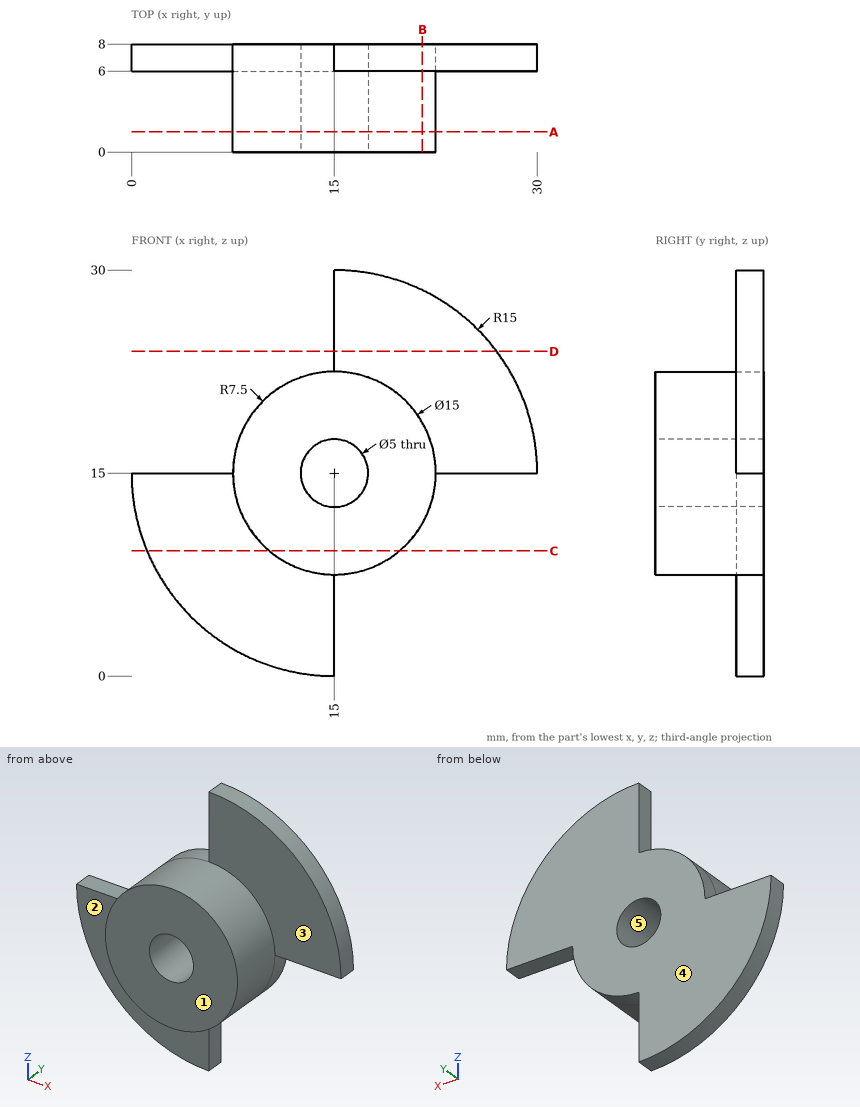
For this review, use the dimensioned drawing (mm, ordinates from the lowest corner) and the shaded views. A direction names the side the tool comes from. Coordinates: 2 decimals unless noted, no trailing zeros. Order: outer loops, then holes, each group sorted by start corner. A loop starts at its lowest first (then second) coordinate and runs counter-clockwise, first axis right, second up. Notation, with made-up numbers: (71.25, -23) - (79.25, -23) arc R26 cw to (79.25, 3) - close; hole circle Ø7 at (-18.75, 6.5). An arc over 180 degrees is marked (long way). Use one line per item in the form item = value.
Q1. For the marked faces 1, 2 and 3, list the 3-axis set-ups (+Z, -Z, +X, -X, +Y, -Y) from which the entire face can be reached by the end or side of a thin tool; tool diameter is ignored.
Checked values:
face_1 = +Z, -Z, +X, -X, -Y
face_2 = -Z, -X, -Y
face_3 = +Z, +X, -Y
Q2. Consider section A-A (y = 1.5). Give the boundary of the cut face in (x, z).
Checked values:
outline = circle Ø15 at (15, 15); hole circle Ø5 at (15, 15)
Q3. For P1, Ø0.6, axis at y = 6.5, z = 2.5, coming from the +X side; P2, Ø1.5, axis at x = 16.5, y = 5.5, coming from the +Z side; P3, Ø1, axis at x = 24, y = 6, coming from the -Z side, all flat-tipped, find the tip position at first contact; note any pin that passes through.
Checked values:
P1 = 15
P2 = 29.97
P3 = 15
Q4. Draft analysis for pull direction X (two halves, no side actions). For the marked faces 4 and 5, state which applies: +X half, -X half, draft (parallel to the pull), parting line (faces both ways), or undercut.
Checked values:
face_4 = draft
face_5 = undercut
Q5. Consider section D-D (z = 24). Give the boundary of the cut face in (x, y).
Checked values:
outline = (15, 6) - (27, 6) - (27, 8) - (15, 8) - close
Q6. Consider section B-B (x = 21.5). Give the boundary of the cut face in (y, z).
Checked values:
outline = (0, 11.26) - (8, 11.26) - (8, 28.52) - (6, 28.52) - (6, 18.74) - (0, 18.74) - close
Q7. For probe 1 along Z at (x, y) = (15, 4.25); probe 2 along Z at (x, y) = (14, 5.75), list the stretches that pass through material, from the lowest coordinate up. Write a range as from..to.
Checked values:
probe_1 = 7.5..12.5, 17.5..22.5
probe_2 = 7.57..12.71, 17.29..22.43
Q8. Consider section C-C (z = 9.25). Give the boundary of the cut face in (x, y), then the cut area to 3 significant figures.
Checked values:
outline = (1.15, 6) - (10.18, 6) - (10.18, 0) - (19.82, 0) - (19.82, 8) - (1.15, 8) - close
area = 95.1 mm2
